Design review of the part built by this model. Coordinates are the model's own, in mm. A direction names the side the tool comes from. Coordinates: 2 decimals unless noted, no trailing zeros. Write each loop counter-clockwise with the first axis right and the second up, starting at its lowest first coordinate (ties: lowest second). Pieces come first, ordered by that corner, then holes.
Q1. For pin 1 Ø10 at (x, z) = (12, 62) entering from +Y; pin 2 Ø10 at (x, y) = (5, -1189) entering from -Z; pin 3 Ø6 at (x, y) = (5, -1619.5) entering from +Z, all flat-tipped, find the tip position at first contact; note any pin that passes through.
Q2. The part is to be moulded in two halves that separate along Y. For faces 1 (the flat face through (10, 99, 1021)), 2 (the flat face through (10, -1504, 629)), 3 (the flat face through (10, -651, 989)), 4 (the flat face through (9.86, -1383.75, 907.06)), say which applies: released by +Y, released by -Y, zero draft, split by the parting line, or undercut.
Q3. Take a section at A-A, the plane z = 391. Write out the cut boundary in (x, y), plus the area to 3 significant figures.
Q4. Take a section at D-D, the plane z = 753. Write out the cut boundary in (x, y).
Q5. For faces 5 (the flat face through (10, -1506, 129)), 6 (the flat face through (10, -1899, 99)), 7 (the flat face through (10, -1346, 174)), list the 3-axis set-ups (+Z, -Z, +X, -X, +Y, -Y) from which the entire face can be reached by the end or side of a thin tool; tool diameter is ignored.
Q6. Take a section at B-B, the plane y = -201.5. Write out the cut boundary in (x, z), plus the area to 3 significant figures.
Q7. Take a section at C-C, the plane x = 12.5. State how many separate pieces and enclosed holes the cut face has, plus the area to 4 significant figures.
Q8. For L1, parallel to Y at x = 7, z = 263; L2, parallel to Z at x = 5, y = -384.5; L3, parallel to Y at x = 9.5, z = 185, list the stretches that pass through material, from the lowest coordinate up.
from build123d import *

# Parameters (mm, degrees)
PAD_DEPTH       = 20
POCKET_DEPTH    = 20
POCKET001_DEPTH = 20
POCKET002_DEPTH = 20


with BuildPart() as part:
    # Sketch → Pad (new body)
    with BuildSketch(Plane.YZ):
        Polygon((-2000, 200), (-2000, 700), (-750, 1120), (0, 1120), (200, 920), (200, 200), (0, 0), (-1800, 0), align=None)
    extrude(amount=PAD_DEPTH)

    # Sketch001 (on Face10 of Pad) → Pocket (cut)
    with BuildSketch(Plane.YZ.offset(20)):
        Polygon((-600, 1040), (-150, 1040), (-50, 940), (-50, 180), (-150, 80), (-600, 80), (-700, 180), (-700, 940), align=None)
    extrude(amount=-POCKET_DEPTH, mode=Mode.SUBTRACT)

    # Sketch002 (on Face5 of Pocket) → Pocket001 (cut)
    with BuildSketch(Plane.YZ.offset(20)):
        Polygon((-1270, 250), (-950, 250), (-800, 100), (-800, 0), (-1420, 0), (-1420, 100), align=None)
    extrude(amount=-POCKET001_DEPTH, mode=Mode.SUBTRACT)

    # Sketch003 (on Face5 of Pocket001) → Pocket002 (cut)
    with BuildSketch(Plane.YZ.offset(20)):
        Polygon((-1755, 80), (-1555, 80), (-1455, 180), (-1455, 580), (-1555, 680), (-1755, 680), (-1855, 580), (-1855, 180), align=None)
    extrude(amount=-POCKET002_DEPTH, mode=Mode.SUBTRACT)


solid = part.part
Responses:
1. pin 1: stops at y = 67
1. pin 2: stops at z = 250
1. pin 3: stops at z = 828.86
2. face 1: released by +Y
2. face 2: undercut
2. face 3: undercut
2. face 4: released by -Y
3. outline: (0, -2000) - (20, -2000) - (20, -1855) - (0, -1855) - close; (0, -1455) - (20, -1455) - (20, -700) - (0, -700) - close; (0, -50) - (20, -50) - (20, 200) - (0, 200) - close
3. area: 23,000 mm2
4. outline: (0, -1842.26) - (20, -1842.26) - (20, -700) - (0, -700) - close; (0, -50) - (20, -50) - (20, 200) - (0, 200) - close
5. face 5: +X, -X
5. face 6: -Z, +X, -X, -Y
5. face 7: -Z, +X, -X
6. outline: (0, 0) - (20, 0) - (20, 80) - (0, 80) - close; (0, 1040) - (20, 1040) - (20, 1120) - (0, 1120) - close
6. area: 3,200 mm2
7. separate pieces: 1
7. enclosed holes: 2
7. area: 1,185,000 mm2
8. L1: y = -2000 to -1855, -1455 to -700, -50 to 200
8. L2: z = 0 to 80, 1040 to 1120
8. L3: y = -1985 to -1855, -1455 to -1335, -885 to -700, -50 to 185
